from build123d import *

# Parameters (mm, degrees)
SKETCH_1_W          = 120
SKETCH_1_H          = 65
EXTRUDE_1_DEPTH     = 5
SKETCH_2_W          = 12.5
SKETCH_2_H          = 12.5
EXTRUDE_2_DEPTH     = 5
SKETCH_3_R          = 3.2
CUT_EXTRUDE_1_DEPTH = 5
SKETCH_4_W          = 3.5
SKETCH_4_H          = 30
EXTRUDE_3_DEPTH     = 9
FILLET_1_R          = 5
FILLET_2_R          = 2.5
SKETCH_5_W          = 25
SKETCH_5_H          = 2.5
EXTRUDE_4_DEPTH     = 6
SKETCH_6_R          = 2
CUT_EXTRUDE_2_DEPTH = 10


with BuildPart() as part:
    # 草图1 → 凸台-拉伸1 (new body)
    with BuildSketch(Plane(origin=(0, 0, 0), x_dir=(1, 0, 0), z_dir=(0, 1, 0))):
        Rectangle(SKETCH_1_W, SKETCH_1_H)
    extrude(amount=EXTRUDE_1_DEPTH)

    # 草图2 → 凸台-拉伸2 (add)
    with BuildSketch(Plane(origin=(0, 5, 0), x_dir=(1, 0, 0), z_dir=(0, 1, 0))):
        with Locations((-36.75, 38.75)):
            Rectangle(SKETCH_2_W, SKETCH_2_H)
        with Locations((36.75, 38.75)):
            Rectangle(SKETCH_2_W, SKETCH_2_H)
        with Locations((36.75, -38.75)):
            Rectangle(SKETCH_2_W, SKETCH_2_H)
        with Locations((-36.75, -38.75)):
            Rectangle(SKETCH_2_W, SKETCH_2_H)
    extrude(amount=-EXTRUDE_2_DEPTH)

    # 草图3 → 切除-拉伸1 (cut)
    with BuildSketch(Plane(origin=(0, 5, 0), x_dir=(1, 0, 0), z_dir=(0, 1, 0))):
        with Locations((-36.75, 38.75)):
            Circle(SKETCH_3_R)
        with Locations((36.75, 38.75)):
            Circle(SKETCH_3_R)
        with Locations((36.75, -38.75)):
            Circle(SKETCH_3_R)
        with Locations((-36.75, -38.75)):
            Circle(SKETCH_3_R)
    extrude(amount=-CUT_EXTRUDE_1_DEPTH, mode=Mode.SUBTRACT)

    # 草图4 → 凸台-拉伸3 (add)
    with BuildSketch(Plane(origin=(0, 5, 0), x_dir=(1, 0, 0), z_dir=(0, 1, 0))):
        with Locations((-58.25, 0)):
            Rectangle(SKETCH_4_W, SKETCH_4_H)
        with Locations((58.25, 0)):
            Rectangle(SKETCH_4_W, SKETCH_4_H)
    extrude(amount=EXTRUDE_3_DEPTH)

    # 圆角1
    fillet_1_edges = [part.edges().sort_by_distance(p)[0] for p in [
        (-43, 2.5, -32.5),
        (-43, 2.5, -45),
        (-30.5, 2.5, -45),
        (-30.5, 2.5, -32.5),
        (43, 2.5, -32.5),
        (30.5, 2.5, -32.5),
        (30.5, 2.5, -45),
        (43, 2.5, -45),
        (30.5, 2.5, 32.5),
        (43, 2.5, 32.5),
        (43, 2.5, 45),
        (30.5, 2.5, 45),
        (-43, 2.5, 32.5),
        (-30.5, 2.5, 32.5),
        (-30.5, 2.5, 45),
        (-43, 2.5, 45),
    ]]
    fillet(fillet_1_edges, radius=FILLET_1_R)

    # 圆角2
    fillet_2_edges = [part.edges().sort_by_distance(p)[0] for p in [
        (60, 2.5, 32.5),
        (-60, 2.5, 32.5),
        (-60, 2.5, -32.5),
        (60, 2.5, -32.5),
    ]]
    fillet(fillet_2_edges, radius=FILLET_2_R)

    # 草图5 → 凸台-拉伸4 (add)
    with BuildSketch(Plane(origin=(0, 5, 0), x_dir=(1, 0, 0), z_dir=(0, 1, 0))):
        with Locations((0, 29.75)):
            Rectangle(SKETCH_5_W, SKETCH_5_H)
        with Locations((0, -29.75)):
            Rectangle(SKETCH_5_W, SKETCH_5_H)
    extrude(amount=EXTRUDE_4_DEPTH)

    # 草图6 → 切除-拉伸2 (cut)
    with BuildSketch(Plane(origin=(0, 5, 0), x_dir=(1, 0, 0), z_dir=(0, 1, 0))):
        with Locations((-56.5, 28.5)):
            Circle(SKETCH_6_R)
        with Locations((56.5, 28.5)):
            Circle(SKETCH_6_R)
        with Locations((56.5, -28.5)):
            Circle(SKETCH_6_R)
        with Locations((-56.5, -28.5)):
            Circle(SKETCH_6_R)
    extrude(amount=-CUT_EXTRUDE_2_DEPTH, mode=Mode.SUBTRACT)


solid = part.part
Geometry check sheet. Reference: the model listing, model coordinates, mm. A direction names the side the tool comes from. Give positions to 0.01 mm unless a question says otherwise; leave off trailing zeros. Loops run counter-clockwise (first coordinate to the right, second up) from the corner with the lowest first, then second, coordinate; pieces in that order, holes last. Notation, with made-up numbers: M 26,30 L 36,30 A15 ccw 36,40 Z; hole C -34.5,-31.5 d4. An arc over 180 degrees is marked long. Answer as a JSON object with one key per item and string values. Group by question number.
Item 1: Sectioned sample at B-B on x = -36.75. Record the boundary of the cut face in (y, z).
Item 2: Material ranges on L1, parallel to X at y = 1.05, z = -38.75; L2, parallel to Z at x = 56.5, y = 4; L3, parallel to Z at x = -36.75, y = 2.4, recorded low to high.
Item 3: Sectioned sample at C-C on z = 13.5. Record the boundary of the cut face in (x, y).
Item 4: Mould release check, pull along Z, two halves, no side actions. Record for faces 6 (the cylindrical face through (56.066, 2.535, 30.452)), 7 (the flat face through (0, 8, 28.5)), 8 (the flat face through (-58, 9, -15)), 9 (the flat face through (-30.5, 3, -39)): pulls with the +Z half, pulls with the -Z half, needs draft (parallel to the pull), parting line crosses it, or undercut.
Item 5: Sectioned sample at D-D on x = 8. Record the boundary of the cut face in (y, z).
Item 6: Gauge pin test, flat ends, axial feed: pin 1 (1.8 mm diameter, centred on x = -5, y = 8, fed in from -Z); pin 2 (5 mm diameter, centred on x = -31, y = 4, fed in from +Z); pin 3 (1.2 mm diameter, centred on y = 2, z = 39, fed in from -X). Record the tip position at first contact, or that the pin passes through.
Item 7: Sectioned sample at A-A on z = -38.75. Record the boundary of the cut face in (x, y).
Item 8: Access from +Z, -Z, +X, -X, +Y, -Y to the whole of each face (thin tool, end or side, straight path). Record for faces 1 (the flat face through (-43, 3, 39)), 2 (the flat face through (30.5, 3, -39)), 3 (the flat face through (-58, 9, 15)), 4 (the flat face through (-43, 3, -39)), 5 (the flat face through (-12.5, 8, -30)).
Findings below:
{
 "1": {"outline": "M 0,-45 L 5,-45 L 5,-41.95 L 0,-41.95 Z; M 0,-35.55 L 5,-35.55 L 5,35.55 L 0,35.55 Z; M 0,41.95 L 5,41.95 L 5,45 L 0,45 Z"},
 "2": {"L1": "-43 to -39.95, -33.55 to -30.5, 30.5 to 33.55, 39.95 to 43", "L2": "-32.5 to -30.5, -26.5 to 26.5, 30.5 to 32.5", "L3": "-45 to -41.95, -35.55 to 35.55, 41.95 to 45"},
 "3": {"outline": "M -60,0 L 60,0 L 60,14 L 56.5,14 L 56.5,5 L -56.5,5 L -56.5,14 L -60,14 Z"},
 "4": {"face 6": "undercut", "face 7": "undercut", "face 8": "pulls with the -Z half", "face 9": "needs draft"},
 "5": {"outline": "M 0,-32.5 L 5,-32.5 L 5,-31 L 11,-31 L 11,-28.5 L 5,-28.5 L 5,28.5 L 11,28.5 L 11,31 L 5,31 L 5,32.5 L 0,32.5 Z"},
 "6": {"pin 1": "z = -31", "pin 2": "z = 44.58", "pin 3": "x = -43"},
 "7": {"outline": "M -43,0 L -39.95,0 L -39.95,5 L -43,5 Z; M -33.55,0 L -30.5,0 L -30.5,5 L -33.55,5 Z; M 30.5,0 L 33.55,0 L 33.55,5 L 30.5,5 Z; M 39.95,0 L 43,0 L 43,5 L 39.95,5 Z"},
 "8": {"face 1": "+Z, -X, +Y, -Y", "face 2": "-Z, +Y, -Y", "face 3": "+Z, +X, -X, +Y", "face 4": "-Z, -X, +Y, -Y", "face 5": "+Z, -Z, -X, +Y"}
}
